Geometry: final body of the model. Coordinates: model frame, mm. A direction names the side the tool comes from. Give positions to 0.01 mm unless a question says otherwise; leave off trailing zeros. Write each loop counter-clockwise with the first axis right and the second up, starting at its lowest first coordinate (ties: lowest second). Pieces come first, ordered by that corner, then holes.
Q1. Mould query, pull axis X, two halves, no side actions, for faces 1 (the cylindrical face through (30.266, -13.289, 3.387)), 2 (the flat face through (-7.74, 14.03, 3.94)), 3 (the flat face through (25, -8.22, 4)). Classes: +X half, -X half, draft (parallel to the pull), parting line (faces both ways), or undercut.
Q2. Section A-A (z = 3). Return the cut outline in (x, y).
Q3. Line query: line 1 (X direction, y = 11, z = 4.75); line 2 (Y direction, x = 25.5, z = 3.5); line 3 (X direction, y = 13, z = 3). Output: solid intervals per line, ascending.
Q4. Section B-B (x = 19.5). Return the cut outline in (y, z).
Q5. Pin query (flat end, axial travel): pin 1 Ø4 at (y, z) = (11.5, 4) entering from +X; pin 2 Ø4 at (y, z) = (-14, 5) entering from +X; pin 3 Ø2.5 at (x, z) = (25.5, 6) entering from +Y. Return the tip coordinate at first contact, or that it passes through.
Q6. Section C-C (y = 0.5). Return the cut outline in (x, z).
Q7. Section D-D (y = -12.5). State how many separate pieces and enclosed holes the cut face has, plus the area to 3 significant figures.
Q8. Reachability of faces 4 (the flat face through (15, 0, 0)), 5 (the flat face through (7.23, 12.326, 3.944)) from +Z, -Z, +X, -X, +Y, -Y: full face, straight path, thin tool, end or side. Return the list, or none.
Autodesk Fusion 360 part; units mm, degrees
sketch "Sketch1" plane through (0, 0, 0) normal (0, 0, 1) x (1, 0, 0)
  line L0 (-0.0194, 16.5) -> (-14.2991, 8.2332)
  line L1 (-14.2991, 8.2332) -> (-14.2797, -8.2668)
  line L2 (-14.2797, -8.2668) -> (0.0194, -16.5)
  line L3 (0.0194, -16.5) -> (14.2991, -8.2332)
  line L4 (14.2991, -8.2332) -> (14.2797, 8.2668)
  line L5 (14.2797, 8.2668) -> (-0.0194, 16.5)
  line L6 (0.2061, 18.4989) -> (-15.9174, 9.4279)
  line L7 (-15.9174, 9.4279) -> (-16.1235, -9.0709)
  line L8 (-16.1235, -9.0709) -> (-0.2061, -18.4989)
  line L9 (-0.2061, -18.4989) -> (15.9174, -9.4279)
  line L10 (15.9174, -9.4279) -> (16.1235, 9.0709)
  line L11 (16.1235, 9.0709) -> (0.2061, 18.4989)
  line L12 (0.2061, 18.4989) -> (35.2061, 18.5399)
  line L13 (35.2061, 18.5399) -> (34.8509, 8.2668)
  line L14 (34.8509, 8.2668) -> (16.1169, 8.4755)
  line L15 (0, 0) -> (14.2894, 0.0168)
  line L16 (-0.2061, -18.4989) -> (34.7939, -18.4989)
  line L17 (34.7939, -18.4989) -> (34.7939, -8.2199)
  line L18 (34.7939, -8.2199) -> (15.9309, -8.2199)
  dimension "d3" = 16.5
  dimension "d4" = 18.5
  dimension "d5" = 35
  dimension "d6" = 35
  dimension "d7" = 10.279
extrude "Extrude1" add sketch "Sketch1" along normal blind 8
sketch "Sketch2" plane through (-0.0217, 18.4986, 0) normal (-0.0012, 1, 0) x (-1, -0.0012, 0)
  line L0 (-35.2278, 0) -> (-0.2278, 0)
  line L1 (-0.2278, 0) -> (-0.2278, 8)
  line L2 (-0.2278, 8) -> (-35.2278, 8)
  line L3 (-35.2278, 8) -> (-35.2278, 0)
  line L4 (-35.2278, 4) -> (-31.7278, 4)
  circle A0 centre (-31.7278, 4) radius 1.6
  dimension "d10" = 3.5
  dimension "d11" = 3.2
extrude "Extrude2" cut sketch "Sketch2" against normal blind 120 contours A0
Computed:
1. face 1: undercut
1. face 2: -X half
1. face 3: draft
2. outline: (-16.12, -9.07) - (-0.21, -18.5) - (30.5, -18.5) - (30.49, -8.22) - (15.93, -8.22) - (16.12, 8.48) - (30.47, 8.32) - (30.46, 18.53) - (0.21, 18.5) - (-15.92, 9.43) - close; (32.96, 18.54) - (32.97, 8.29) - (34.85, 8.27) - (35.21, 18.54) - close; (32.99, -8.22) - (33, -18.5) - (34.79, -18.5) - (34.79, -8.22) - close; hole (-14.3, 8.23) - (-14.28, -8.27) - (0.02, -16.5) - (14.3, -8.23) - (14.28, 8.27) - (-0.02, 16.5) - close
3. line 1: x = -13.12 to -9.52, 9.53 to 30.3, 33.13 to 34.95
3. line 2: y = -18.5 to -8.22, 8.37 to 18.53
3. line 3: x = -9.57 to -6.07, 6.06 to 30.46, 32.96 to 35.01
4. outline: (-18.5, 0) - (-8.22, 0) - (-8.22, 8) - (-18.5, 8) - close; (8.44, 0) - (18.52, 0) - (18.52, 8) - (8.44, 8) - close
5. pin 1: stops at x = 35.03
5. pin 2: stops at x = 34.79
5. pin 3: stops at y = 18.53
6. outline: (-16.02, 0) - (-14.29, 0) - (-14.29, 8) - (-16.02, 8) - close; (14.29, 0) - (16.03, 0) - (16.03, 8) - (14.29, 8) - close
7. separate pieces: 2
7. enclosed holes: 1
7. area: 242 mm2
8. face 4: -Z, +X, -X, +Y, -Y
8. face 5: +Z, -Z
